CAD build for the part. Positions are in the model's coordinates, mm. Face numbers are marked on the shaded views. A direction names the side the tool comes from. Round coordinates to 2 decimals unless told otherwise and drop trailing zeros. Write each loop counter-clockwise with the first axis right and the second up, starting at its lowest first coordinate (ties: lowest second). Pieces come first, ordered by that corner, then holes. Notation, with made-up numbers: (26, 71) - (76, 71) arc R10 cw to (76, 84) - close; hole circle Ø10 at (8, 22.25). An arc over 180 degrees is marked (long way). Answer in a Markdown table with one row per item.
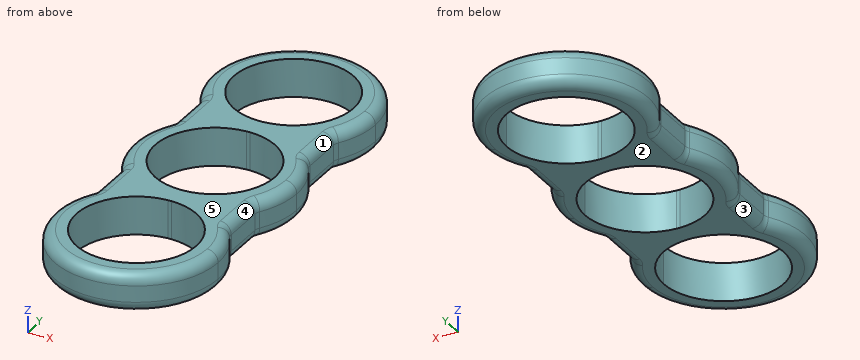
```python
from build123d import *

# Parameters (mm, degrees)
F1_DEPTH = 7
F2_F1_R  = 2
F2_F2_R  = 2


with BuildPart() as f1:
    # F0 (on Top) → F1 (new body)
    with BuildSketch(Plane.XY):
        with BuildLine():
            ThreePointArc((0.3357339129, 14.9962422873), (4.0392104898, 14.4459260215), (7.4910247439, 12.9955587909))
            ThreePointArc((7.4910247439, 12.9955587909), (10.1759290258, 14.9706607644), (12.3583803583, 17.4899156126))
            ThreePointArc((12.3583803583, 17.4899156126), (14.3243796615, 21.540033746), (15, 25.9911175817))
            ThreePointArc((15, 25.9911175817), (-4.4510838357, 40.3154972432), (-12.3583803583, 17.4899156126))
            ThreePointArc((-12.3583803583, 17.4899156126), (-10.1759290258, 14.9706607644), (-7.4910247439, 12.9955587909))
            ThreePointArc((-7.4910247439, 12.9955587909), (-4.0392104898, 14.4459260215), (-0.3357339129, 14.9962422873))
            ThreePointArc((-0.3357339129, 14.9962422873), (-7.6585549211, 33.8870998842), (11, 25.9911175817))
            ThreePointArc((11, 25.9911175817), (7.8959823025, 18.3325626607), (0.3357339129, 14.9962422873))
        make_face()
        with BuildLine():
            ThreePointArc((-0.3357339129, 10.9948752944), (0, 11), (0.3357339129, 10.9948752944))
            ThreePointArc((0.3357339129, 10.9948752944), (4.0392104898, 11.5451915602), (7.4910247439, 12.9955587909))
            ThreePointArc((7.4910247439, 12.9955587909), (4.0392104898, 14.4459260215), (0.3357339129, 14.9962422873))
            ThreePointArc((0.3357339129, 14.9962422873), (0, 14.9911175817), (-0.3357339129, 14.9962422873))
            ThreePointArc((-0.3357339129, 14.9962422873), (-4.0392104898, 14.4459260215), (-7.4910247439, 12.9955587909))
            ThreePointArc((-7.4910247439, 12.9955587909), (-4.0392104898, 11.5451915602), (-0.3357339129, 10.9948752944))
        make_face()
        with BuildLine():
            ThreePointArc((12.3583803583, 17.4899156126), (10.1759290258, 14.9706607644), (7.4910247439, 12.9955587909))
            ThreePointArc((7.4910247439, 12.9955587909), (10.1759290258, 11.0204568173), (12.3583803583, 8.5012019691))
            Line((12.3583803583, 8.5012019691), (12.3583803583, 17.4899156126))
        make_face()
        with BuildLine():
            ThreePointArc((-12.3583803583, 8.5012019691), (-10.1759290258, 11.0204568173), (-7.4910247439, 12.9955587909))
            ThreePointArc((-7.4910247439, 12.9955587909), (-10.1759290258, 14.9706607644), (-12.3583803583, 17.4899156126))
            Line((-12.3583803583, 17.4899156126), (-12.3583803583, 8.5012019691))
        make_face()
        with BuildLine():
            ThreePointArc((-0.3357339129, -10.9948752944), (-11, 0), (-0.3357339129, 10.9948752944))
            ThreePointArc((-0.3357339129, 10.9948752944), (-4.0392104898, 11.5451915602), (-7.4910247439, 12.9955587909))
            ThreePointArc((-7.4910247439, 12.9955587909), (-10.1759290258, 11.0204568173), (-12.3583803583, 8.5012019691))
            ThreePointArc((-12.3583803583, 8.5012019691), (-15, 0), (-12.3583803583, -8.5012019691))
            ThreePointArc((-12.3583803583, -8.5012019691), (-10.1759290258, -11.0204568173), (-7.4910247439, -12.9955587909))
            ThreePointArc((-7.4910247439, -12.9955587909), (-4.0392104898, -11.5451915602), (-0.3357339129, -10.9948752944))
        make_face()
        with BuildLine():
            ThreePointArc((12.3583803583, -8.5012019691), (10.1759290258, -11.0204568173), (7.4910247439, -12.9955587909))
            ThreePointArc((7.4910247439, -12.9955587909), (10.1759290258, -14.9706607644), (12.3583803583, -17.4899156126))
            Line((12.3583803583, -17.4899156126), (12.3583803583, -8.5012019691))
        make_face()
        with BuildLine():
            ThreePointArc((-12.3583803583, -17.4899156126), (-10.1759290258, -14.9706607644), (-7.4910247439, -12.9955587909))
            ThreePointArc((-7.4910247439, -12.9955587909), (-10.1759290258, -11.0204568173), (-12.3583803583, -8.5012019691))
            Line((-12.3583803583, -8.5012019691), (-12.3583803583, -17.4899156126))
        make_face()
        with BuildLine():
            ThreePointArc((7.4910247439, -12.9955587909), (4.0392104898, -11.5451915602), (0.3357339129, -10.9948752944))
            ThreePointArc((0.3357339129, -10.9948752944), (0, -11), (-0.3357339129, -10.9948752944))
            ThreePointArc((-0.3357339129, -10.9948752944), (-4.0392104898, -11.5451915602), (-7.4910247439, -12.9955587909))
            ThreePointArc((-7.4910247439, -12.9955587909), (-4.0392104898, -14.4459260215), (-0.3357339129, -14.9962422873))
            ThreePointArc((-0.3357339129, -14.9962422873), (0, -14.9911175817), (0.3357339129, -14.9962422873))
            ThreePointArc((0.3357339129, -14.9962422873), (4.0392104898, -14.4459260215), (7.4910247439, -12.9955587909))
        make_face()
        with BuildLine():
            ThreePointArc((12.3583803583, -17.4899156126), (10.1759290258, -14.9706607644), (7.4910247439, -12.9955587909))
            ThreePointArc((7.4910247439, -12.9955587909), (4.0392104898, -14.4459260215), (0.3357339129, -14.9962422873))
            ThreePointArc((0.3357339129, -14.9962422873), (7.8959823025, -18.3325626607), (11, -25.9911175817))
            ThreePointArc((11, -25.9911175817), (-7.6585549211, -33.8870998842), (-0.3357339129, -14.9962422873))
            ThreePointArc((-0.3357339129, -14.9962422873), (-4.0392104898, -14.4459260215), (-7.4910247439, -12.9955587909))
            ThreePointArc((-7.4910247439, -12.9955587909), (-10.1759290258, -14.9706607644), (-12.3583803583, -17.4899156126))
            ThreePointArc((-12.3583803583, -17.4899156126), (-4.4510838357, -40.3154972432), (15, -25.9911175817))
            ThreePointArc((15, -25.9911175817), (14.3243796615, -21.540033746), (12.3583803583, -17.4899156126))
        make_face()
        with BuildLine():
            ThreePointArc((0.3357339129, 10.9948752944), (7.8959823025, 7.6585549211), (11, 0))
            ThreePointArc((11, 0), (7.8959823025, -7.6585549211), (0.3357339129, -10.9948752944))
            ThreePointArc((0.3357339129, -10.9948752944), (4.0392104898, -11.5451915602), (7.4910247439, -12.9955587909))
            ThreePointArc((7.4910247439, -12.9955587909), (10.1759290258, -11.0204568173), (12.3583803583, -8.5012019691))
            ThreePointArc((12.3583803583, -8.5012019691), (14.3243796615, -4.4510838357), (15, 0))
            ThreePointArc((15, 0), (14.3243796615, 4.4510838357), (12.3583803583, 8.5012019691))
            ThreePointArc((12.3583803583, 8.5012019691), (10.1759290258, 11.0204568173), (7.4910247439, 12.9955587909))
            ThreePointArc((7.4910247439, 12.9955587909), (4.0392104898, 11.5451915602), (0.3357339129, 10.9948752944))
        make_face()
    extrude(amount=F1_DEPTH)

    # F2: fillet of radius 2 on 16 edges, made by hand

    # F2_f1
    f2_f1_edges = [f1.edges().sort_by_distance(p)[0] for p in [
        (-12.3583803583, -17.4899156126, 3.5),
        (12.3583803583, -17.4899156126, 3.5),
        (12.3583803583, -8.5012019691, 3.5),
        (12.3583803583, 8.5012019691, 3.5),
        (12.3583803583, 17.4899156126, 3.5),
        (-12.3583803583, 17.4899156126, 3.5),
        (-12.3583803583, 8.5012019691, 3.5),
        (-12.3583803583, -8.5012019691, 3.5),
    ]]
    fillet(f2_f1_edges, radius=F2_F1_R)

    # F2_f2
    f2_f2_edges = [f1.edges().sort_by_distance(p)[0] for p in [
        (0, -40.9911175817, 0),
        (0, -40.9911175817, 7),
        (15, 0, 0),
        (15, 0, 7),
        (0, 40.9911175817, 0),
        (0, 40.9911175817, 7),
        (-15, 0, 0),
        (-15, 0, 7),
        (-12.4376458065, 8.5440032789, 7),
        (-12.4376458065, -8.5440032789, 7),
        (-12.4376458065, 8.5440032789, 0),
        (-12.4376458065, -8.5440032789, 0),
        (12.4376458065, 17.4471143028, 7),
        (-12.4376458065, 17.4471143028, 7),
        (12.4376458065, 17.4471143028, 0),
        (-12.4376458065, 17.4471143028, 0),
        (12.4376458065, -8.5440032789, 7),
        (12.4376458065, 8.5440032789, 7),
        (12.4376458065, -8.5440032789, 0),
        (12.4376458065, 8.5440032789, 0),
        (-12.4376458065, -17.4471143028, 7),
        (12.4376458065, -17.4471143028, 7),
        (-12.4376458065, -17.4471143028, 0),
        (12.4376458065, -17.4471143028, 0),
    ]]
    fillet(f2_f2_edges, radius=F2_F2_R)


solid = f1.part
```
Q1. Saw through at A-A on z = 3.5. List the corners of the cut face in (x, y), then the cut area to 3 significant figures.
Computed:
| item | result |
|---|---|
| outline | (-12.67, -17.96) arc R15 ccw (long way) to (12.67, -17.96) arc R2 cw to (12.36, -16.89) - (12.36, -9.1) arc R2 cw to (12.67, -8.03) arc R15 ccw to (12.67, 8.03) arc R2 cw to (12.36, 9.1) - (12.36, 16.89) arc R2 cw to (12.67, 17.96) arc R15 ccw (long way) to (-12.67, 17.96) arc R2 cw to (-12.36, 16.89) - (-12.36, 9.1) arc R2 cw to (-12.67, 8.03) arc R15 ccw to (-12.67, -8.03) arc R2 cw to (-12.36, -9.1) - (-12.36, -16.89) arc R2 cw to start; hole circle Ø22 at (0, -25.99); hole circle Ø22 at (0, 0); hole circle Ø22 at (0, 25.99) |
| area | 974 mm2 |
Q2. 3-axis set-ups, long thin cutter, end or side, ignore diameter. For the marked faces 1, 2 and 3: which of +Z, -Z, +X, -X, +Y, -Y reach the whole face in a straight line?
Computed:
| item | result |
|---|---|
| face 1 | +Z, +X |
| face 2 | -Z, +X, -X, +Y, -Y |
| face 3 | -Z, -X |
Q3. Drill centre lines: line 1 (Y direction, x = 0, z = 3); line 2 (X direction, y = -7.5, z = 2); line 3 (Y direction, x = 0, z = 1.5). Where is each one in solid material? Low to high.
Computed:
| item | result |
|---|---|
| line 1 | y = -40.99 to -36.99, -14.99 to -11, 11 to 14.99, 36.99 to 40.99 |
| line 2 | x = -12.99 to -8.05, 8.05 to 12.99 |
| line 3 | y = -40.93 to -36.99, -14.99 to -11, 11 to 14.99, 36.99 to 40.93 |
Q4. Flat gauge pins, fed straight in: pin 1 (1.5 mm diameter, centred on y = 13.5, z = 3, fed in from -X); pin 2 (2 mm diameter, centred on y = -31.5, z = 3.5, fed in from -X); pin 3 (2.5 mm diameter, centred on y = 12, z = 3, fed in from +X). Where does each tip first touch, or does it go through?
Computed:
| item | result |
|---|---|
| pin 1 | stops at x = -12.36 |
| pin 2 | stops at x = -14.31 |
| pin 3 | stops at x = 12.36 |
Q5. Pull direction Y, two halves, no side cores. Call the marked faces 4 and 5: released by +Y, released by -Y, zero draft, split by the parting line, or undercut.
Computed:
| item | result |
|---|---|
| face 4 | undercut |
| face 5 | zero draft |
Q6. Saw through at B-B on x = 8. Count the separate pieces of the cut face and the enclosed holes in it, then the cut area to 3 significant figures.
Computed:
| item | result |
|---|---|
| separate pieces | 4 |
| enclosed holes | 0 |
| area | 220 mm2 |
